For this review, take the finished solid that the model builds, in its own axes (mm). Face numbers are marked on the shaded views. A direction names the side the tool comes from. Give positions to 0.01 mm unless a question says otherwise; leave off trailing zeros. Write each loop counter-clockwise with the first axis right and the second up, starting at its lowest first coordinate (ties: lowest second). Pieces come first, ordered by that corner, then holes.
Q1. We need section B-B (x = 25.25). Write out the cut boundary in (y, z).
Q2. For line 1 (Z direction, x = 0.6, y = 25.6); line 2 (X direction, y = 5, z = 12.75), list the stretches that pass through material, from the lowest coordinate up.
Q3. Insertion check: P1, Ø4, axis at x = 17.5, z = 13, coming from the +Y side; P2, Ø1, axis at y = 23, z = 9, coming from the +X side; P3, Ø2, axis at x = 25.5, z = 9.5, coming from the -Y side; P4, Ø3.5, axis at x = 16.71, z = 20, coming from the +Y side. Each pin has a flat end and moves straight along its axis. Give the tip position at first contact, or say it passes through.
Q4. Machinability: for the marked faces 1 and 2, which of the approach directions +Z, -Z, +X, -X, +Y, -Y give a long, thin tool a straight path to every point of the face, cutting with its end or side? Answer none if there is none.
Q5. We need section D-D (y = 5). Write out the cut boundary in (x, z).
Q6. We need section C-C (z = 11.5). Give the number of separate pieces and of enclosed holes in the cut face, then the cut area to 3 significant figures.
Q7. We need section A-A (z = 5). Write out the cut boundary in (x, y).
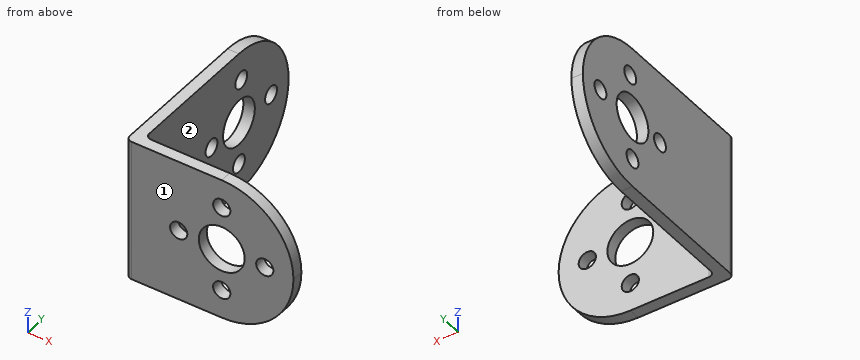
```python
from build123d import *

# Parameters (mm, degrees)
SKETCH1_W           = 27.21
SKETCH1_H           = 2
BOSS_EXTRUDE1_DEPTH = 25
SKETCH2_R           = 1.5
SKETCH2_R_2         = 4
CUT_EXTRUDE1_DEPTH  = 25
SKETCH3_R           = 1.5
SKETCH3_R_2         = 4
CUT_EXTRUDE3_DEPTH  = 25
FILLET1_R           = 1


with BuildPart() as part:
    # Sketch1 → Boss-Extrude1 (new body)
    with BuildSketch(Plane.XY):
        Polygon((2, 2), (2, 38.1), (0, 38.1), (0, 0), (2, 0), align=None)
        with Locations((15.605, 1)):
            Rectangle(SKETCH1_W, SKETCH1_H)
    extrude(amount=BOSS_EXTRUDE1_DEPTH)

    # Sketch2 → Cut-Extrude1 (cut)
    with BuildSketch(Plane(origin=(0, 2, 0), x_dir=(1, 0, 0), z_dir=(0, 1, 0))):
        with Locations(Location((16.71, -20, 0), (0, 0, 270))):
            Circle(SKETCH2_R)
        with Locations(Location((9.21, -12.5, 0), (0, 0, 270))):
            Circle(SKETCH2_R)
        with Locations(Location((16.71, -5, 0), (0, 0, 270))):
            Circle(SKETCH2_R)
        with Locations(Location((24.21, -12.5, 0), (0, 0, 270))):
            Circle(SKETCH2_R)
        with Locations(Location((16.71, -12.5, 0), (0, 0, 270))):
            Circle(SKETCH2_R_2)
        with BuildLine():
            Line((29.21, -12.5), (29.21, 0))
            Line((29.21, 0), (16.71, 0))
            ThreePointArc((16.71, 0), (25.548834765, -3.661165235), (29.21, -12.5))
        make_face()
        with BuildLine():
            Line((29.21, -25), (29.21, -12.5))
            ThreePointArc((29.21, -12.5), (25.548834765, -21.338834765), (16.71, -25))
            Line((16.71, -25), (29.21, -25))
        make_face()
    extrude(amount=-CUT_EXTRUDE1_DEPTH, mode=Mode.SUBTRACT)

    # Sketch3 → Cut-Extrude3 (cut)
    with BuildSketch(Plane(origin=(2, 0, 0), x_dir=(0, 0, -1), z_dir=(1, 0, 0))):
        with BuildLine():
            ThreePointArc((-25, 25.599999976), (-21.338834773, 34.438834756), (-12.5, 38.1))
            Line((-12.5, 38.1), (-25, 38.1))
            Line((-25, 38.1), (-25, 25.599999976))
        make_face()
        with BuildLine():
            Line((0, 25.6), (0, 38.1))
            Line((0, 38.1), (-12.5, 38.1))
            ThreePointArc((-12.5, 38.1), (-3.661165235, 34.438834765), (0, 25.6))
        make_face()
        with Locations(Location((-12.390951319, 33.683987084, 0), (0, 0, 90))):
            Circle(SKETCH3_R)
        with Locations(Location((-5, 25.6, 0), (0, 0, 90))):
            Circle(SKETCH3_R)
        with Locations(Location((-19.890951319, 26.183987084, 0), (0, 0, 90))):
            Circle(SKETCH3_R)
        with Locations(Location((-12.5, 25.6, 0), (0, 0, 90))):
            Circle(SKETCH3_R_2)
        with Locations(Location((-12.390951319, 18.683987084, 0), (0, 0, 90))):
            Circle(SKETCH3_R)
    extrude(amount=-CUT_EXTRUDE3_DEPTH, mode=Mode.SUBTRACT)

    # Fillet1
    fillet1_edges = [part.edges().sort_by_distance(p)[0] for p in [
        (2, 2, 12.5),
        (0, 0, 12.5),
    ]]
    fillet(fillet1_edges, radius=FILLET1_R)


solid = part.part
```
Computed:
1. outline: (0, 3.37) - (2, 3.37) - (2, 11.42) - (0, 11.42) - close; (0, 13.58) - (2, 13.58) - (2, 21.63) - (0, 21.63) - close
2. line 1: z = 0 to 3.5, 6.5 to 8.5, 16.5 to 18.51, 21.27 to 25
2. line 2: x = 0 to 2
3. P1: passes through
3. P2: stops at x = 2
3. P3: stops at y = 0
3. P4: stops at y = 2
4. face 1: +Z, -Z, +X, -X, -Y
4. face 2: +Z, -Z, +X, +Y
5. outline: (0, 0) - (2, 0) - (2, 25) - (0, 25) - close
6. separate pieces: 7
6. enclosed holes: 0
6. area: 80.9 mm2
7. outline: (0, 1) arc R1 ccw to (1, 0) - (15.21, 0) - (15.21, 2) - (3, 2) arc R1 cw to (2, 3) - (2, 24.1) - (0, 24.1) - close; (0, 27.1) - (2, 27.1) - (2, 35.6) - (0, 35.6) - close; (18.21, 0) - (26.71, 0) - (26.71, 2) - (18.21, 2) - close
